The listing builds one solid part. Answer for the finished solid, in the listing's coordinates (mm). Coordinates: 2 decimals unless noted, no trailing zeros. Order: outer loops, then holes, each group sorted by start corner. A loop starts at its lowest first (then second) coordinate and runs counter-clockwise, first axis right, second up. Notation, with made-up numbers: (-18, 80) - (37, 80) arc R18 cw to (37, 106) - close; hole circle Ø5 at (60, -24). An arc over 180 degrees is marked (long way). Use a Markdown table: item, result. Add a question column.
Item 1: The part is cut by section B-B, the plane y = -6.25. Give the vertices of the cut face in (x, z), then the cut area to 3 significant figures.
Item 2: Find the intervals of material crossed by line 1 along X through (y, z) = (4.5, 6.5); line 2 along Y through (x, z) = (10, 9); line 3 along Y through (x, z) = (-7, 28), in increasing order.
Item 3: The part is cut by section C-C, the plane x = -7.5. Give the vertices of the cut face in (y, z).
Item 4: A flat-ended cylindrical pin translates along its axis: P1, Ø3, axis at x = -9, y = -1, coming from the +Z side. Find the tip coordinate at first contact, or state that the pin passes through.
Item 5: The part is cut by section D-D, the plane y = 8.75. Give the vertices of the cut face in (x, z).
Item 6: The part is cut by section A-A, the plane x = 14. Give the vertices of the cut face in (y, z).
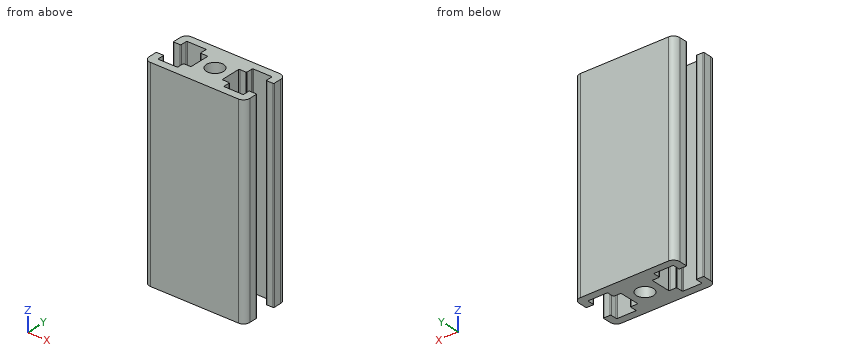
from build123d import *

# Parameters (mm, degrees)
SKETCH_1_R      = 3.4
EXTRUDE_1_DEPTH = 80


with BuildPart() as part:
    # 草图1 → 凸台-拉伸1 (new body)
    with BuildSketch(Plane.XY):
        with BuildLine():
            Line((20.229808423, 4.055287365), (20.229808423, 7.155287365))
            ThreePointArc((20.229808423, 7.155287365), (19.497575376, 8.923054318), (17.729808423, 9.655287365))
            Line((17.729808423, 9.655287365), (-17.270191577, 9.655287365))
            ThreePointArc((-17.270191577, 9.655287365), (-19.03795853, 8.923054318), (-19.770191577, 7.155287365))
            Line((-19.770191577, 7.155287365), (-19.770191577, 4.055287365))
            ThreePointArc((-19.770191577, 4.055287365), (-19.682323611, 3.843155331), (-19.470191577, 3.755287365))
            Line((-19.470191577, 3.755287365), (-17.070191577, 3.755287365))
            ThreePointArc((-17.070191577, 3.755287365), (-16.858059542, 3.843155331), (-16.770191577, 4.055287365))
            Line((-16.770191577, 4.055287365), (-16.770191577, 6.355287365))
            ThreePointArc((-16.770191577, 6.355287365), (-16.682323611, 6.567419399), (-16.470191577, 6.655287365))
            Line((-16.470191577, 6.655287365), (-9.270191577, 6.655287365))
            ThreePointArc((-9.270191577, 6.655287365), (-9.058059542, 6.567419399), (-8.970191577, 6.355287365))
            Line((-8.970191577, 6.355287365), (-8.970191577, 4.055287365))
            ThreePointArc((-8.970191577, 4.055287365), (-8.882323611, 3.843155331), (-8.670191577, 3.755287365))
            Line((-8.670191577, 3.755287365), (-6.270191577, 3.755287365))
            ThreePointArc((-6.270191577, 3.755287365), (-6.058059542, 3.667419399), (-5.970191577, 3.455287365))
            Line((-5.970191577, 3.455287365), (-5.970191577, -4.144712635))
            ThreePointArc((-5.970191577, -4.144712635), (-6.058059542, -4.356844669), (-6.270191577, -4.444712635))
            Line((-6.270191577, -4.444712635), (-8.670191577, -4.444712635))
            ThreePointArc((-8.670191577, -4.444712635), (-8.882323611, -4.532580601), (-8.970191577, -4.744712635))
            Line((-8.970191577, -4.744712635), (-8.970191577, -7.044712635))
            ThreePointArc((-8.970191577, -7.044712635), (-9.058059542, -7.256844669), (-9.270191577, -7.344712635))
            Line((-9.270191577, -7.344712635), (-16.470191577, -7.344712635))
            ThreePointArc((-16.470191577, -7.344712635), (-16.682323611, -7.256844669), (-16.770191577, -7.044712635))
            Line((-16.770191577, -7.044712635), (-16.770191577, -4.744712635))
            ThreePointArc((-16.770191577, -4.744712635), (-16.858059542, -4.532580601), (-17.070191577, -4.444712635))
            Line((-17.070191577, -4.444712635), (-19.470191577, -4.444712635))
            ThreePointArc((-19.470191577, -4.444712635), (-19.682323611, -4.532580601), (-19.770191577, -4.744712635))
            Line((-19.770191577, -4.744712635), (-19.770191577, -7.844712635))
            ThreePointArc((-19.770191577, -7.844712635), (-19.03795853, -9.612479588), (-17.270191577, -10.344712635))
            Line((-17.270191577, -10.344712635), (17.729808423, -10.344712635))
            ThreePointArc((17.729808423, -10.344712635), (19.497575376, -9.612479588), (20.229808423, -7.844712635))
            Line((20.229808423, -7.844712635), (20.229808423, -4.744712635))
            ThreePointArc((20.229808423, -4.744712635), (20.141940458, -4.532580601), (19.929808423, -4.444712635))
            Line((19.929808423, -4.444712635), (17.529808423, -4.444712635))
            ThreePointArc((17.529808423, -4.444712635), (17.317676389, -4.532580601), (17.229808423, -4.744712635))
            Line((17.229808423, -4.744712635), (17.229808423, -7.044712635))
            ThreePointArc((17.229808423, -7.044712635), (17.141940458, -7.256844669), (16.929808423, -7.344712635))
            Line((16.929808423, -7.344712635), (9.729808423, -7.344712635))
            ThreePointArc((9.729808423, -7.344712635), (9.517676389, -7.256844669), (9.429808423, -7.044712635))
            Line((9.429808423, -7.044712635), (9.429808423, -4.744712635))
            ThreePointArc((9.429808423, -4.744712635), (9.341940458, -4.532580601), (9.129808423, -4.444712635))
            Line((9.129808423, -4.444712635), (6.729808423, -4.444712635))
            ThreePointArc((6.729808423, -4.444712635), (6.517676389, -4.356844669), (6.429808423, -4.144712635))
            Line((6.429808423, -4.144712635), (6.429808423, 3.455287365))
            ThreePointArc((6.429808423, 3.455287365), (6.517676389, 3.667419399), (6.729808423, 3.755287365))
            Line((6.729808423, 3.755287365), (9.129808423, 3.755287365))
            ThreePointArc((9.129808423, 3.755287365), (9.341940458, 3.843155331), (9.429808423, 4.055287365))
            Line((9.429808423, 4.055287365), (9.429808423, 6.355287365))
            ThreePointArc((9.429808423, 6.355287365), (9.517676389, 6.567419399), (9.729808423, 6.655287365))
            Line((9.729808423, 6.655287365), (16.929808423, 6.655287365))
            ThreePointArc((16.929808423, 6.655287365), (17.141940458, 6.567419399), (17.229808423, 6.355287365))
            Line((17.229808423, 6.355287365), (17.229808423, 4.055287365))
            ThreePointArc((17.229808423, 4.055287365), (17.317676389, 3.843155331), (17.529808423, 3.755287365))
            Line((17.529808423, 3.755287365), (19.929808423, 3.755287365))
            ThreePointArc((19.929808423, 3.755287365), (20.141940458, 3.843155331), (20.229808423, 4.055287365))
        make_face()
        with Locations((0.229808423, -0.344712635)):
            Circle(SKETCH_1_R, mode=Mode.SUBTRACT)
    extrude(amount=EXTRUDE_1_DEPTH)


solid = part.part
Solution:
| question | item | result |
|---|---|---|
| 1 | outline | (-19.77, 0) - (-16.77, 0) - (-16.77, 80) - (-19.77, 80) - close; (-8.97, 0) - (9.43, 0) - (9.43, 80) - (-8.97, 80) - close; (17.23, 0) - (20.23, 0) - (20.23, 80) - (17.23, 80) - close |
| 1 | area | 1,950 mm2 |
| 2 | line 1 | x = -19.77 to -16.77, -8.97 to 9.43, 17.23 to 20.23 |
| 2 | line 2 | y = -10.34 to -7.34, 6.66 to 9.66 |
| 2 | line 3 | y = -10.34 to -4.44, 3.76 to 9.66 |
| 3 | outline | (-10.34, 0) - (-4.44, 0) - (-4.44, 80) - (-10.34, 80) - close; (3.76, 0) - (9.66, 0) - (9.66, 80) - (3.76, 80) - close |
| 4 | P1 | passes through |
| 5 | outline | (-19.2, 0) - (19.66, 0) - (19.66, 80) - (-19.2, 80) - close |
| 6 | outline | (-10.34, 0) - (-7.34, 0) - (-7.34, 80) - (-10.34, 80) - close; (6.66, 0) - (9.66, 0) - (9.66, 80) - (6.66, 80) - close |
